```python
from build123d import *

# Parameters (mm, degrees)
BOSS_EXTRUDE1_DEPTH = 10
SKETCH2_W           = 30
SKETCH2_H           = 10
BOSS_EXTRUDE2_DEPTH = 7.5
CUT_EXTRUDE1_REACH  = 12
SKETCH3_W           = 4
SKETCH3_H           = 21


with BuildPart() as part:
    # Sketch1 → Boss-Extrude1 (new body)
    with BuildSketch(Plane(origin=(0, 0, -10.04783639), x_dir=(-1, 0, 0), z_dir=(0, 0, -1))):
        Polygon((24.605530087, 10.619804964), (22.967664033, 6.119804964), (22.371275694, 6.119804964), (22.371275694, -1.380195036), (72.371275694, -1.380195036), (72.371275694, 6.119804964), (71.509404954, 6.119804964), (69.8715389, 10.619804964), (68.587827187, 10.619804964), (66.949961133, 6.119804964), (65.226219654, 6.119804964), (63.5883536, 10.619804964), (62.304641887, 10.619804964), (60.666775833, 6.119804964), (58.943034354, 6.119804964), (57.3051683, 10.619804964), (56.021456587, 10.619804964), (54.383590533, 6.119804964), (52.659849054, 6.119804964), (51.021983, 10.619804964), (49.738271287, 10.619804964), (48.100405233, 6.119804964), (46.376663754, 6.119804964), (44.7387977, 10.619804964), (43.455085987, 10.619804964), (41.817219933, 6.119804964), (40.093478454, 6.119804964), (38.4556124, 10.619804964), (37.171900687, 10.619804964), (35.534034633, 6.119804964), (33.810293154, 6.119804964), (32.1724271, 10.619804964), (30.888715387, 10.619804964), (29.250849333, 6.119804964), (27.527107854, 6.119804964), (25.8892418, 10.619804964), align=None)
    extrude(amount=-BOSS_EXTRUDE1_DEPTH)

    # Sketch2 → Boss-Extrude2 (add)
    with BuildSketch(Plane(origin=(-22.371275694, 0, 0), x_dir=(0, 0, -1), z_dir=(1, 0, 0))):
        with Locations((5.04783639, 2.369804964)):
            Rectangle(SKETCH2_W, SKETCH2_H)
    extrude(amount=BOSS_EXTRUDE2_DEPTH)

    # Sketch3 → Cut-Extrude1 (cut, up to next)
    with BuildSketch(Plane(origin=(0, 7.369804964, 0), x_dir=(-1, 0, 0), z_dir=(0, 1, 0)), mode=Mode.PRIVATE) as cut_extrude1_sk1:
        with Locations((18.621275694, -5.04783639)):
            Rectangle(SKETCH3_W, SKETCH3_H)
    cut_extrude1_tool1 = extrude(cut_extrude1_sk1.sketch, amount=-CUT_EXTRUDE1_REACH, mode=Mode.PRIVATE) & part.part
    add(cut_extrude1_tool1.solids().sort_by_distance((-18.621276, 7.369805, -5.047836))[0], mode=Mode.SUBTRACT)


solid = part.part
```
Model file for the job. Use its own axes, mm. A direction names the side the tool comes from. Give positions to 0.01 mm unless a question says otherwise; leave off trailing zeros. Loops run counter-clockwise (first coordinate to the right, second up) from the corner with the lowest first, then second, coordinate; pieces in that order, holes last. Notation, with made-up numbers: (44, 48) -> (85, 48) arc R8 ccw to (85, 61) -> close; hole circle Ø8 at (-39.75, -26.5). An arc over 180 degrees is marked (long way). Write each question's results on one line, items separated by ' | '.
(1) Cut at D-D on y = 9.5. Give the number of separate pieces and of enclosed holes in the cut face, and give its area (3 significant figures).
Geometry results:
separate pieces: 8 | enclosed holes: 0 | area: 168 mm²
(2) Tool access for faces 3 (the flat face through (-47, -1.38, -5)), 4 (the flat face through (-44, 10.62, -5)), 5 (the flat face through (-47, 6.12, -5)), 6 (the flat face through (-21, -2.63, -5)), 7 (the flat face through (-20.621, 2, -5)): list every direction of +Z, -Z, +X, -X, +Y, -Y with a clear straight run to the whole face (end or side of a thin tool).
Geometry results:
face 3: +Z, -Z, -X, -Y | face 4: +Z, -Z, +X, -X, +Y | face 5: +Z, -Z, +Y | face 6: +Z, -Z, +X, -X, -Y | face 7: +Y, -Y
(3) Pull direction X, two halves, no side cores. Call faces 1 (the flat face through (-57, 10.62, -5)), 2 (the flat face through (-51.85, 8.34, -5.12)): released by +X, released by -X, zero draft, split by the parting line, or undercut.
Geometry results:
face 1: zero draft | face 2: undercut
(4) Flat gauge pins, fed straight in: pin 1 Ø1 at (y, z) = (6, -14) entering from -X; pin 2 Ø3.5 at (x, y) = (-36.5, 4.5) entering from +Z; pin 3 Ø1.4 at (x, z) = (-66, -6.5) entering from +Y. Where does each tip first touch, or does it go through?
Geometry results:
pin 1: stops at x = -22.37 | pin 2: stops at z = -0.05 | pin 3: stops at y = 6.12
(5) Cut at C-C on x = -20. List the corners of the cut face in (y, z), and give its area (3 significant figures).
Geometry results:
outline: (-2.63, -20.05) -> (7.37, -20.05) -> (7.37, -15.55) -> (-2.63, -15.55) -> close; (-2.63, 5.45) -> (7.37, 5.45) -> (7.37, 9.95) -> (-2.63, 9.95) -> close | area: 90.0 mm²
(6) Cut at B-B on y = 0.75. List the corners of the cut face in (x, z).
Geometry results:
outline: (-72.37, -10.05) -> (-22.37, -10.05) -> (-22.37, -20.05) -> (-14.87, -20.05) -> (-14.87, 9.95) -> (-22.37, 9.95) -> (-22.37, -0.05) -> (-72.37, -0.05) -> close; hole (-20.62, -15.55) -> (-16.62, -15.55) -> (-16.62, 5.45) -> (-20.62, 5.45) -> close
(7) Probe line 1 along X through (y, z) = (2, -15); line 2 along X through (y, z) = (4, -9.5); line 3 along Z through (x, y) = (-17.5, -1.75). List the from-to ranges inside material, lowest first.
Geometry results:
line 1: x = -22.37 to -20.62, -16.62 to -14.87 | line 2: x = -72.37 to -20.62, -16.62 to -14.87 | line 3: z = -20.05 to -15.55, 5.45 to 9.95
(8) Cut at A-A on z = -13.5. List the corners of the cut face in (x, y).
Geometry results:
outline: (-22.37, -2.63) -> (-20.62, -2.63) -> (-20.62, 7.37) -> (-22.37, 7.37) -> close; (-16.62, -2.63) -> (-14.87, -2.63) -> (-14.87, 7.37) -> (-16.62, 7.37) -> close
